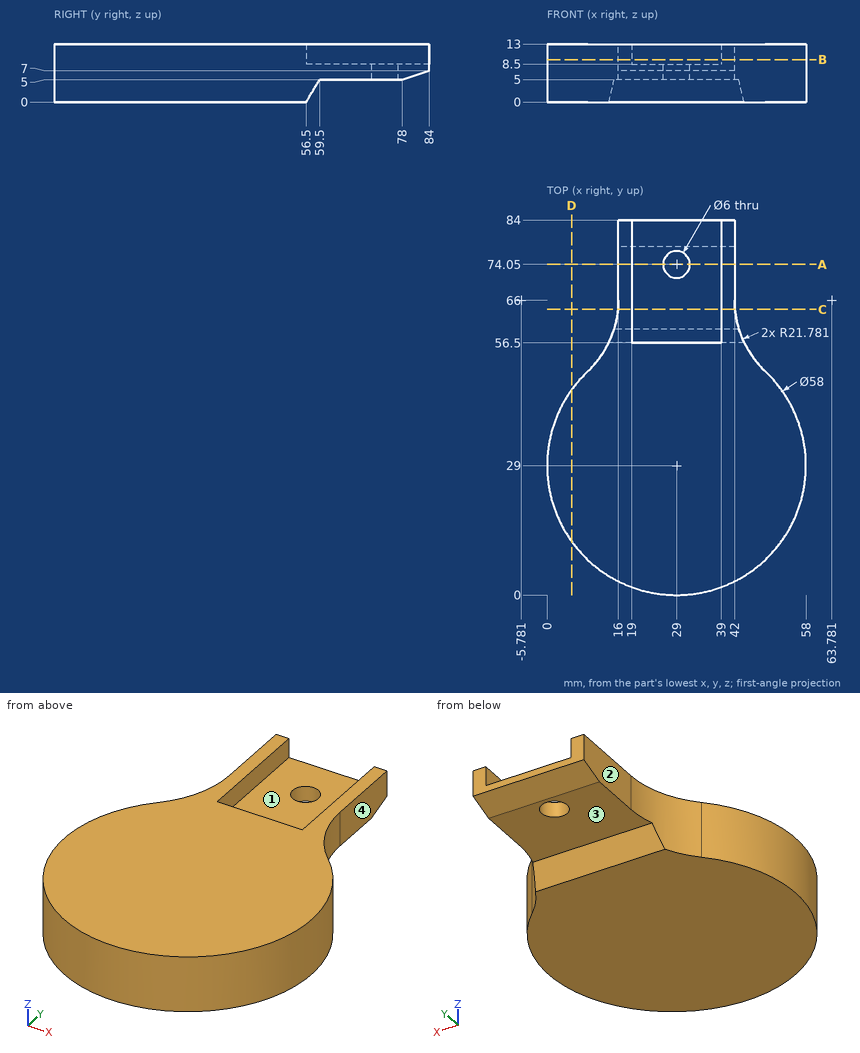
Geometry: see drawing. Coordinates: mm, zero at the bounding-box minimum. A direction names the side the tool comes from. Round coordinates to 2 decimals unless told otherwise and drop trailing zeros. Order: outer loops, then holes, each group sorted by start corner. A loop starts at its lowest first (then second) coordinate and runs counter-clockwise, first axis right, second up. Notation, with made-up numbers: (-1.75, 15) - (20.25, 15) arc R26 ccw to (20.25, 52) - close; hole circle Ø3 at (-35, -13.75). An arc over 180 degrees is marked (long way). Use a Markdown table: item, result. Add a question column.
1. Line query: probe 1 along X at (y, z) = (77, 11); probe 2 along Y at (x, z) = (29, 7.7); probe 3 along X at (y, z) = (74.05, 5.8). Output: solid intervals per line, ascending.
2. First-contact query: pin 1 (4 mm diameter, centred on y = 24, z = 3, fed in from -X); pin 2 (1.3 mm diameter, centred on y = 66.5, z = 10.5, fed in from +X); pin 3 (10 mm diameter, centred on x = 31.5, y = 70, fed in from +Z). Flat tips, straight axial feed; report the tip coordinate or a pass-through.
3. Set-up query: the marked faces 1, 2, 3 and 4. Return all of +Z, -Z, +X, -X, +Y, -Y with unobstructed straight access to the full face (end or side cutting, diameter ignored); none if empty.
4. Section query A-A (y = 74.05). Return the cut outline in (x, z).
5. Section query B-B (z = 9.5). Return the cut outline in (x, y).
6. Section query C-C (y = 64). Return the cut outline in (x, z).
7. Section query D-D (x = 5.5). Return the cut outline in (y, z), then the cut area to 3 significant figures.
Derived:
| question | item | result |
|---|---|---|
| 1 | probe 1 | 16 to 19, 39 to 42 |
| 1 | probe 2 | 0 to 71.05, 77.05 to 84 |
| 1 | probe 3 | 16 to 26, 32 to 42 |
| 2 | pin 1 | x = 0.16 |
| 2 | pin 2 | x = 42 |
| 2 | pin 3 | z = 8.5 |
| 3 | face 1 | +Z, +Y |
| 3 | face 2 | +Z, -Z, -X, +Y |
| 3 | face 3 | -Z, +X, -X, +Y |
| 3 | face 4 | +Z, -Z, +X, +Y |
| 4 | outline | (16, 5) - (26, 5) - (26, 8.5) - (19, 8.5) - (19, 13) - (16, 13) - close; (32, 5) - (42, 5) - (42, 13) - (39, 13) - (39, 8.5) - (32, 8.5) - close |
| 5 | outline | (9.14, 50.13) arc R29 ccw (long way) to (48.86, 50.13) arc R21.78 cw to (42, 66) - (42, 84) - (39, 84) - (39, 56.5) - (19, 56.5) - (19, 84) - (16, 84) - (16, 66) arc R21.78 cw to start |
| 6 | outline | (15.91, 5) - (42.09, 5) - (42.09, 13) - (39, 13) - (39, 8.5) - (19, 8.5) - (19, 13) - (15.91, 13) - close |
| 7 | outline | (12.01, 0) - (45.99, 0) - (45.99, 13) - (12.01, 13) - close |
| 7 | area | 442 mm2 |
